from build123d import *

# Parameters (mm, degrees)
SKETCH1_R                  = 1.75
BASE_FLANGE1_DEPTH         = 2
SKETCHED_START             = -8.2
SKETCHED_BEND1_DEPTH       = 15.2
SKETCHED_BEND1_2_DEPTH     = 8.4499999
SKETCHED_START_2           = 3.7500001
SKETCHED_BEND1_3_DEPTH     = 3.2499999
SKETCHED_START_3           = 0.2499999
SKETCHED_BEND1_4_DEPTH     = 3.5000002
SKETCHED_START_4           = -12.7366
SKETCHED_BEND1_5_OUTLINE_R = 1.75
SKETCHED_BEND1_5_DEPTH     = 25.4732
SKETCH7_R                  = 37
CUT_EXTRUDE1_DEPTH         = 20.330576261
BOSS_EXTRUDE1_DEPTH        = 2


with BuildPart() as part:
    # Base-Flange1: sheet metal written as solids
    # Sketch1 → Base-Flange1 (new body)
    with BuildSketch(Plane.XY):
        with BuildLine():
            Line((10, 7), (22, 7))
            Line((22, 7), (22, -8.2))
            Line((22, -8.2), (10, -8.2))
            Line((10, -8.2), (10, -7))
            ThreePointArc((10, -7), (0, -5.623026261), (-10, -7))
            Line((-10, -7), (-10, -8.2))
            Line((-10, -8.2), (-22, -8.2))
            Line((-22, -8.2), (-22, 7))
            Line((-22, 7), (-10, 7))
            Line((-10, 7), (10, 7))
        make_face()
        with Locations((18, 2)):
            Circle(SKETCH1_R, mode=Mode.SUBTRACT)
        with Locations(Location((-18, 2, 0), (0, 0, 180))):
            Circle(SKETCH1_R, mode=Mode.SUBTRACT)
    extrude(amount=-BASE_FLANGE1_DEPTH)

    # Sketched Bend1: read off the stored shape, not the designer's step
    # Sketched Bend1 outline → Sketched Bend1 (cut)
    with BuildSketch(Plane(origin=(0, 0, 0), x_dir=(1, 0, 0), z_dir=(0, 1, 0)).offset(SKETCHED_START)):
        with BuildLine():
            ThreePointArc((-10, 0), (-11.654267209, 0.556604688), (-12.635602398, 2))
            Line((-12.635602398, 2), (-22, 2))
            Line((-22, 2), (-22, 0))
            Line((-22, 0), (-10, 0))
        make_face()
        with BuildLine():
            Line((22, 2), (12.635602398, 2))
            ThreePointArc((12.635602398, 2), (11.654267209, 0.556604688), (10, 0))
            Line((10, 0), (22, 0))
            Line((22, 0), (22, 2))
        make_face()
    extrude(amount=SKETCHED_BEND1_DEPTH, mode=Mode.SUBTRACT)

    # Sketched Bend1 2 outline → Sketched Bend1 2 (add)
    with BuildSketch(Plane(origin=(0, 0, 0), x_dir=(1, 0, 0), z_dir=(0, 1, 0)).offset(SKETCHED_START)):
        with BuildLine():
            ThreePointArc((-10, 2), (-10.520854855, 2.215745145), (-10.7366, 2.7366))
            Line((-10.7366, 2.7366), (-10.7366, 12.008755099))
            Line((-10.7366, 12.008755099), (-12.7366, 12.008755099))
            Line((-12.7366, 12.008755099), (-12.7366, 2.7366))
            ThreePointArc((-12.7366, 2.7366), (-12.711233029, 2.364854094), (-12.635602398, 2))
            Line((-12.635602398, 2), (-10, 2))
        make_face()
        with BuildLine():
            ThreePointArc((10.7366, 2.7366), (10.520854855, 2.215745145), (10, 2))
            Line((10, 2), (12.635602398, 2))
            ThreePointArc((12.635602398, 2), (12.711233029, 2.364854094), (12.7366, 2.7366))
            Line((12.7366, 2.7366), (12.7366, 12.008755099))
            Line((12.7366, 12.008755099), (10.7366, 12.008755099))
            Line((10.7366, 12.008755099), (10.7366, 2.7366))
        make_face()
    extrude(amount=SKETCHED_BEND1_2_DEPTH)

    # Sketched Bend1 3 outline → Sketched Bend1 3 (add)
    with BuildSketch(Plane(origin=(0, 0, 0), x_dir=(1, 0, 0), z_dir=(0, 1, 0)).offset(SKETCHED_START_2)):
        with BuildLine():
            ThreePointArc((-10, 2), (-10.520854855, 2.215745145), (-10.7366, 2.7366))
            Line((-10.7366, 2.7366), (-10.7366, 12.008755099))
            Line((-10.7366, 12.008755099), (-12.7366, 12.008755099))
            Line((-12.7366, 12.008755099), (-12.7366, 2.7366))
            ThreePointArc((-12.7366, 2.7366), (-12.711233029, 2.364854094), (-12.635602398, 2))
            Line((-12.635602398, 2), (-10, 2))
        make_face()
        with BuildLine():
            ThreePointArc((10.7366, 2.7366), (10.520854855, 2.215745145), (10, 2))
            Line((10, 2), (12.635602398, 2))
            ThreePointArc((12.635602398, 2), (12.711233029, 2.364854094), (12.7366, 2.7366))
            Line((12.7366, 2.7366), (12.7366, 12.008755099))
            Line((12.7366, 12.008755099), (10.7366, 12.008755099))
            Line((10.7366, 12.008755099), (10.7366, 2.7366))
        make_face()
    extrude(amount=SKETCHED_BEND1_3_DEPTH)

    # Sketched Bend1 4 outline → Sketched Bend1 4 (add)
    with BuildSketch(Plane(origin=(0, 0, 0), x_dir=(1, 0, 0), z_dir=(0, 1, 0)).offset(SKETCHED_START_3)):
        with BuildLine():
            ThreePointArc((10.7366, 2.7366), (10.520854855, 2.215745145), (10, 2))
            Line((10, 2), (12.635602398, 2))
            ThreePointArc((12.635602398, 2), (12.711233029, 2.364854094), (12.7366, 2.7366))
            Line((12.7366, 2.7366), (12.7366, 12.008755099))
            Line((12.7366, 12.008755099), (10.7366, 12.008755099))
            Line((10.7366, 12.008755099), (10.7366, 2.7366))
        make_face()
        with BuildLine():
            ThreePointArc((-10, 2), (-10.520854855, 2.215745145), (-10.7366, 2.7366))
            Line((-10.7366, 2.7366), (-10.7366, 12.008755099))
            Line((-10.7366, 12.008755099), (-12.7366, 12.008755099))
            Line((-12.7366, 12.008755099), (-12.7366, 2.7366))
            ThreePointArc((-12.7366, 2.7366), (-12.711233029, 2.364854094), (-12.635602398, 2))
            Line((-12.635602398, 2), (-10, 2))
        make_face()
    extrude(amount=SKETCHED_BEND1_4_DEPTH)

    # Sketched Bend1 5 outline → Sketched Bend1 5 (cut)
    with BuildSketch(Plane.YZ.offset(SKETCHED_START_4)):
        with Locations((2, -8.008755099)):
            Circle(SKETCHED_BEND1_5_OUTLINE_R)
    extrude(amount=SKETCHED_BEND1_5_DEPTH, mode=Mode.SUBTRACT)

    # Sketch7 → Cut-Extrude1 (cut, through all)
    with BuildSketch(Plane.XY):
        with Locations((0, -42.623026261)):
            Circle(SKETCH7_R)
    extrude(amount=-CUT_EXTRUDE1_DEPTH, mode=Mode.SUBTRACT)

    # Sketch8 → Boss-Extrude1 (add)
    with BuildSketch(Plane(origin=(0, 0, -12.008755099), x_dir=(-1, 0, 0), z_dir=(0, 0, -1))):
        with BuildLine():
            Line((-12.7366, -7.884301177), (-12.7366, 7))
            Line((-12.7366, 7), (12.7366, 7))
            Line((12.7366, 7), (12.7366, -7.884301177))
            ThreePointArc((12.7366, -7.884301177), (0, -5.623026261), (-12.7366, -7.884301177))
        make_face()
    extrude(amount=BOSS_EXTRUDE1_DEPTH)


solid = part.part
Could you check a few things on this model? Use its own coordinates, in mm. A direction names the side the tool comes from. Coordinates: 2 decimals unless noted, no trailing zeros. Loops run counter-clockwise (first coordinate to the right, second up) from the corner with the lowest first, then second, coordinate; pieces in that order, holes last.
1. Imagine slicing it at A-A (z = -5.25). Please give me the cut outline in (x, y), and give its area (3 significant figures).
2. Imagine slicing it at D-D (z = -7). Please give me the cut outline in (x, y).
3. For P1, Ø3, axis at y = 2, z = -8.01, coming from the -X side, with a flat end and sliding along its axis, tell me the tip position at first contact or that it passes through.
4. I need wall thicknesses on L1, parallel to X at y = -5, z = -3.5; L2, parallel to Z at x = 3.25, y = 4.75; L3, parallel to Z at x = 12.2, y = 2. Which ranges of each line are inside material? Lowest first, please.
5. We'd pull the mould along X, two halves only. Please class faces 3 (the face through (-12.737, 0, -8)), 4 (the face through (12.737, -1, -8)), 5 (the face through (0, 0, -2)): released by +X, released by -X, zero draft, split by the parting line, or undercut.
6. Imagine slicing it at C-C (y = -4.25). Please give me the cut outline in (x, z).
7. Imagine slicing it at B-B (y = 2). Please give me the cut outline in (x, z), and give its area (3 significant figures).
8. For faces 1 (the face through (0, 0, -12.009)), 2 (the face through (11.723, 3.617, -8.679)), which set-ups out of +Z, -Z, +X, -X, +Y, -Y let a thin tool reach every point of the face, with its end or its side?
Computed values:
1. outline: (-12.74, -7.88) arc R37 cw to (-10.74, -7.22) - (-10.74, 7) - (-12.74, 7) - close; (10.74, -7.22) arc R37 cw to (12.74, -7.88) - (12.74, 7) - (10.74, 7) - close
1. area: 58.2 mm2
2. outline: (-12.74, -7.88) arc R37 cw to (-10.74, -7.22) - (-10.74, 0.57) - (-12.74, 0.57) - close; (-12.74, 3.43) - (-10.74, 3.43) - (-10.74, 7) - (-12.74, 7) - close; (10.74, -7.22) arc R37 cw to (12.74, -7.88) - (12.74, 0.57) - (10.74, 0.57) - close; (10.74, 3.43) - (12.74, 3.43) - (12.74, 7) - (10.74, 7) - close
3. P1: passes through
4. L1: x = -12.74 to -10.74, 10.74 to 12.74
4. L2: z = -14.01 to -12.01, -2 to 0
4. L3: z = -14.01 to -9.76, -6.26 to -1.11
5. face 3: released by -X
5. face 4: released by +X
5. face 5: undercut
6. outline: (-12.74, -14.01) - (12.74, -14.01) - (12.74, -2.74) arc R2.74 ccw to (10, 0) - (-10, 0) arc R2.74 ccw to (-12.74, -2.74) - close; hole (-10.74, -12.01) - (10.74, -12.01) - (10.74, -2.74) arc R0.74 ccw to (10, -2) - (-10, -2) arc R0.74 ccw to (-10.74, -2.74) - close
7. outline: (-12.74, -14.01) - (12.74, -14.01) - (12.74, -9.76) - (10.74, -9.76) - (10.74, -12.01) - (-10.74, -12.01) - (-10.74, -9.76) - (-12.74, -9.76) - close; (-12.74, -6.26) - (-10.74, -6.26) - (-10.74, -2.74) arc R0.74 cw to (-10, -2) - (10, -2) arc R0.74 cw to (10.74, -2.74) - (10.74, -6.26) - (12.74, -6.26) - (12.74, -2.74) arc R2.74 ccw to (10, 0) - (-10, 0) arc R2.74 ccw to (-12.74, -2.74) - close
7. area: 125 mm2
8. face 1: +Y, -Y
8. face 2: +X, -X
